```python
from build123d import *

# Parameters (mm, degrees)
SALIENTE_EXTRUIR1_DEPTH = 80
CROQUIS2_R              = 39
CORTAR_EXTRUIR1_DEPTH   = 1
CROQUIS3_R              = 2.5
CORTAR_EXTRUIR2_DEPTH   = 6
CROQUIS5_R              = 1.5
CORTAR_EXTRUIR3_DEPTH   = 40


with BuildPart() as part:
    # Croquis1 → Saliente-Extruir1 (new body)
    with BuildSketch(Plane.XY):
        Polygon((-50, 0), (50, 0), (-50, 26.794919243), align=None)
    extrude(amount=SALIENTE_EXTRUIR1_DEPTH)

    # Croquis2 → Cortar-Extruir1 (cut)
    with BuildSketch(Plane(origin=(3.349364905, 12.5, 0), x_dir=(0.96592582628907, -0.2588190451025143, 0), z_dir=(0.2588190451025143, 0.96592582628907, 0))):
        with Locations(Location((-6.231326727, -40, 0), (0, 0, 180))):
            Circle(CROQUIS2_R)
    extrude(amount=-CORTAR_EXTRUIR1_DEPTH, mode=Mode.SUBTRACT)

    # Croquis3 → Cortar-Extruir2 (cut)
    with BuildSketch(Plane(origin=(3.09054586, 11.534074174, 0), x_dir=(0.96592582628907, -0.2588190451025143, 0), z_dir=(0.2588190451025143, 0.96592582628907, 0))):
        with Locations(Location((-6.231326727, -9, 0), (0, 0, 180))):
            Circle(CROQUIS3_R)
        with Locations(Location((-6.231326727, -71, 0), (0, 0, 180))):
            Circle(CROQUIS3_R)
    extrude(amount=-CORTAR_EXTRUIR2_DEPTH, mode=Mode.SUBTRACT)

    # Croquis5 → Cortar-Extruir3 (cut)
    with BuildSketch(Plane.XZ):
        with Locations(Location((-45, 75, 0), (0, 0, 270))):
            Circle(CROQUIS5_R)
        with Locations((45, 75)):
            Circle(CROQUIS5_R)
        with Locations(Location((45, 5, 0), (0, 0, 270))):
            Circle(CROQUIS5_R)
        with Locations((-45, 5)):
            Circle(CROQUIS5_R)
    extrude(amount=-CORTAR_EXTRUIR3_DEPTH, mode=Mode.SUBTRACT)


solid = part.part
```
Geometry: final body of the model. Coordinates: model frame, mm. A direction names the side the tool comes from. Coordinates: 2 decimals unless noted, no trailing zeros. Order: outer loops, then holes, each group sorted by start corner. A loop starts at its lowest first (then second) coordinate and runs counter-clockwise, first axis right, second up. Notation, with made-up numbers: (65, 57.25) -> (73, 57.25) arc R14 ccw to (73, 63.25) -> close; hole circle Ø4 at (-1.5, 42.25). An arc over 180 degrees is marked (long way). Write each question's results on one line, items separated by ' | '. Start each with the question number.
1) Cut plane D-D, the plane y = 21.5. State how many separate pieces and enclosed holes the cut face has, and give its area (3 significant figures).
2) Cut plane A-A, the plane x = -45. Output: boundary loops of the cut face in (y, z), and give its area (3 significant figures).
3) Mould query, pull axis X, two halves, no side actions, for faces 3 (the flat face through (-23, 8, 0)), 4 (the flat face through (-50, 14, 39)), 5 (the cylindrical face through (-46.5, 12.77, 5.07)), 6 (the cylindrical face through (-3.17, 10.15, 68.56)). Classes: released by +X, released by -X, zero draft, split by the parting line, or undercut.
4) Material intervals for line 1 along Z through (x, y) = (-45, 11.5); line 2 along Z through (x, y) = (-3.5, 11.5); line 3 along X through (y, z) = (1.1, 75), sorted ascending.
5) Set-up query: faces 1 (the flat face through (-4.448, 7.342, 9.035)), 2 (the flat face through (-23, 8, 80)). Return all of +Z, -Z, +X, -X, +Y, -Y with unobstructed straight access to the full face (end or side cutting, diameter ignored); none if empty.
6) Cut plane B-B, the plane z = 5. Output: boundary loops of the cut face in (x, y).
7) Cut plane C-C, the plane z = 58. Output: boundary loops of the cut face in (x, y).
8) First-contact query: pin 1 (6 mm diameter, centred on x = -25.5, z = 49, fed in from +Y). Flat tip, straight axial feed; report the tip coordinate or a pass-through.
Checks:
1) separate pieces: 1 | enclosed holes: 2 | area: 1,380 mm^2
2) outline: (0, 0) -> (25.46, 0) -> (25.46, 3.5) -> (0, 3.5) -> close; (0, 6.5) -> (25.46, 6.5) -> (25.46, 73.5) -> (0, 73.5) -> close; (0, 76.5) -> (25.46, 76.5) -> (25.46, 80) -> (0, 80) -> close | area: 1,880 mm^2
3) face 3: zero draft | face 4: released by -X | face 5: undercut | face 6: undercut
4) line 1: 0 to 3.5, 6.5 to 73.5, 76.5 to 80 | line 2: 0 to 6.5, 11.5 to 68.5, 73.5 to 80 | line 3: -50 to -46.5, -43.5 to 43.5
5) face 1: none | face 2: +Z, +X, -X, +Y, -Y
6) outline: (-50, 0) -> (-46.5, 0) -> (-46.5, 25.86) -> (-50, 26.79) -> close; (-43.5, 0) -> (43.5, 0) -> (43.5, 1.74) -> (13.95, 9.66) -> (13.69, 8.69) -> (-19.55, 17.6) -> (-19.29, 18.57) -> (-43.5, 25.05) -> close; (46.5, 0) -> (50, 0) -> (46.5, 0.94) -> close
7) outline: (-50, 0) -> (50, 0) -> (30.75, 5.16) -> (30.49, 4.19) -> (-36.35, 22.1) -> (-36.09, 23.07) -> (-50, 26.79) -> close
8) pin 1: y = 20
